Part model, mm, in its own coordinate system. A direction names the side the tool comes from. Give positions to 0.01 mm unless a question says otherwise; leave off trailing zeros. Write each loop counter-clockwise with the first axis right and the second up, starting at its lowest first coordinate (ties: lowest second). Pieces come first, ordered by that corner, then holes. Notation, with made-up numbers: (49, 2.25) - (84, 2.25) arc R30 ccw to (84, 36.25) - close; hole circle Ø1 at (1.25, 32.25). An arc over 180 degrees is marked (long way). Answer in a Markdown table with one row per item. Add a question column.
1. Drop flat-ended pins along their axis: pin 1 Ø8 at (x, z) = (-146.5, 3.5) entering from +Y; pin 2 Ø1.5 at (y, z) = (-78, 6.5) entering from +X; pin 3 Ø4 at (x, z) = (-67.5, 7.5) entering from +Y. Give the stop position or say it passes through.
2. Band-saw the part on D-D on z = 9.25. State how many separate pieces and enclosed holes the cut face has, plus the area to 3 significant figures.
3. Pull direction Y, two halves, no side cores. Call faces 4 (the flat face through (-30, -152, 4)), 5 (the cylindrical face through (-125.45, -108.18, 5.92)), 6 (the flat face through (-126, -175, 4)): released by +Y, released by -Y, zero draft, split by the parting line, or undercut.
4. Band-saw the part on A-A on y = -144.5. Write the cut outline in (x, z), plus the area to 3 significant figures.
5. Band-saw the part on B-B on x = -212.5. Write the cut outline in (y, z).
6. Band-saw the part on C-C on y = -162.5. Write the cut outline in (x, z).
7. Which spindle directions (+Z, -Z, +X, -X, +Y, -Y) get a long thin tool onto all of the face, cutting with end or side? Do faces 1 (the flat face through (-40, -144, 6)), 2 (the flat face through (-121, -99, 0)), 3 (the flat face through (-199, -30, 4)). Say none if no direction does.
8. Probe line 1 along X through (y, z) = (-162.5, 7); line 2 along X through (y, z) = (-144, 10.5); line 3 along Y through (x, z) = (-199, 11). List the from-to ranges inside material, lowest first.
```python
from build123d import *

# Parameters (mm, degrees)
F1_DEPTH  = 12
F2_W      = 200
F2_H      = 20
F3_DEPTH  = 5
F4_W      = 155
F4_H      = 20
F5_DEPTH  = 5
F6_R      = 2.5
F7_DEPTH  = 25
F9_DEPTH  = 5
F10_W     = 195
F10_H     = 30
F10_W_2   = 30
F10_H_2   = 145
F11_DEPTH = 25
F12_W     = 145
F12_H     = 9
F13_DEPTH = 195.0010001
F15_DEPTH = 25


with BuildPart() as f1:
    # F0 (on Top) → F1 (new body)
    with BuildSketch(Plane.XY):
        with BuildLine():
            add(Edge.make_bspline(
                [(-176, 0), (-176, -130), (0, -130)],
                knots=[3.1415926536, 3.1415926536, 3.1415926536, 4.7123889804, 4.7123889804, 4.7123889804], degree=2, weights=[1, 0.7071067812, 1]))
            Line((-176, 0), (-176, -130))
            Line((-176, -130), (0, -130))
        make_face()
        Polygon((-176, -130), (-176, 0), (-200, 0), (-200, -150), (0, -150), (0, -130), align=None)
    extrude(amount=F1_DEPTH)

    # F2 (on face) → F3 (join)
    with BuildSketch(Plane.XZ.offset(150)):
        with Locations((-100, 6)):
            Rectangle(F2_W, F2_H)
    extrude(amount=F3_DEPTH)

    # F4 (on face) → F5 (join)
    with BuildSketch(Plane(origin=(-200, 0, 0), x_dir=(0, -1, 0), z_dir=(-1, 0, 0))):
        with Locations((77.5, 6)):
            Rectangle(F4_W, F4_H)
    extrude(amount=F5_DEPTH)

    # F6 (on face) → F7 (join)
    with BuildSketch(Plane(origin=(0, 0, -4), x_dir=(1, 0, 0), z_dir=(0, 0, -1))):
        Polygon((0, 155), (0, 175), (-225, 175), (-225, 0), (-205, 0), (-205, 155), align=None)
        with Locations((-212.5, 60)):
            Circle(F6_R, mode=Mode.SUBTRACT)
        with Locations((-212.5, 115)):
            Circle(F6_R, mode=Mode.SUBTRACT)
        with Locations((-165, 162.5)):
            Circle(F6_R, mode=Mode.SUBTRACT)
        with Locations((-60, 162.5)):
            Circle(F6_R, mode=Mode.SUBTRACT)
    extrude(amount=-F7_DEPTH)

    # F8 (on face) → F9 (join)
    with BuildSketch(Plane.XY.offset(16)):
        Polygon((-190, 0), (-205, 0), (-205, -155), (0, -155), (0, -140), (-190, -140), align=None)
    extrude(amount=F9_DEPTH)

    # F10 (on Top) → F11 (cut, symmetric)
    with BuildSketch(Plane.XY):
        with Locations((-127.5, -15)):
            Rectangle(F10_W, F10_H)
        with Locations((-15, -15)):
            Rectangle(F10_W_2, F10_H)
        with Locations((-15, -102.5)):
            Rectangle(F10_W_2, F10_H_2)
    extrude(amount=F11_DEPTH, both=True, mode=Mode.SUBTRACT)

    # F12 (on face) → F13 (cut, through all)
    with BuildSketch(Plane.YZ.offset(-30)):
        with Locations((-102.5, 16.5)):
            Rectangle(F12_W, F12_H)
    extrude(amount=-F13_DEPTH, mode=Mode.SUBTRACT)

    # F14 (on face) → F15 (cut)
    with BuildSketch(Plane(origin=(0, 0, 0), x_dir=(1, 0, 0), z_dir=(0, 0, -1))):
        with BuildLine():
            ThreePointArc((-181.2494979045, 40), (-124.4154289012, 108.9058025162), (-40, 138.0975202339))
            Line((-40, 138.0975202339), (-40, 150))
            Line((-40, 150), (-200, 150))
            Line((-200, 150), (-200, 40))
            Line((-200, 40), (-181.2494979045, 40))
        make_face()
    extrude(amount=-F15_DEPTH, mode=Mode.SUBTRACT)


solid = f1.part
```
Values:
| question | item | result |
|---|---|---|
| 1 | pin 1 | stops at y = -67.4 |
| 1 | pin 2 | stops at x = -140.03 |
| 1 | pin 3 | stops at y = -119.43 |
| 2 | separate pieces | 1 |
| 2 | enclosed holes | 5 |
| 2 | area | 10,600 mm² |
| 3 | face 4 | zero draft |
| 3 | face 5 | undercut |
| 3 | face 6 | released by -Y |
| 4 | outline | (-225, -4) - (-200, -4) - (-200, 12) - (-225, 12) - close; (-40, 0) - (-30, 0) - (-30, 12) - (-40, 12) - close |
| 4 | area | 520 mm² |
| 5 | outline | (-175, -4) - (-117.5, -4) - (-117.5, 12) - (-175, 12) - close; (-112.5, -4) - (-62.5, -4) - (-62.5, 12) - (-112.5, 12) - close; (-57.5, -4) - (-30, -4) - (-30, 12) - (-57.5, 12) - close |
| 6 | outline | (-225, -4) - (-167.5, -4) - (-167.5, 12) - (-225, 12) - close; (-162.5, -4) - (-62.5, -4) - (-62.5, 12) - (-162.5, 12) - close; (-57.5, -4) - (-30, -4) - (-30, 12) - (-57.5, 12) - close |
| 7 | face 1 | +Z, -Z |
| 7 | face 2 | -Z, +X, +Y |
| 7 | face 3 | +Z, -Z, +X, -X, +Y |
| 8 | line 1 | x = -225 to -167.5, -162.5 to -62.5, -57.5 to -30 |
| 8 | line 2 | x = -225 to -200, -40 to -30 |
| 8 | line 3 | y = -175 to -150, -40 to -30 |
